The model under review builds one solid part; all positions refer to its coordinate system, in mm. A direction names the side the tool comes from. Give positions to 0.01 mm unless a question says otherwise; leave off trailing zeros. Write each loop counter-clockwise with the first axis right and the second up, starting at its lowest first coordinate (ties: lowest second). Pieces come first, ordered by that corner, then holes. Notation, with made-up numbers: M 86.5,80 L 99.5,80 A17 cw 99.5,105 Z; hole C -15,83 d5. An arc over 180 degrees is marked long. Write each question's results on one line, items separated by ' | '. Start each with the question number.
from build123d import *

# Parameters (mm, degrees)
F0_W     = 112.393752
F0_H     = 112.393752
F1_DEPTH = 50
F2_R     = 20
F3_DEPTH = 30
F2_R_2   = 30
F4_DEPTH = 20


with BuildPart() as f1:
    # F0 (on Top) → F1 (new body)
    with BuildSketch(Plane.XY):
        Rectangle(F0_W, F0_H)
    extrude(amount=F1_DEPTH)

    # F2 (on face) → F3 (cut)
    with BuildSketch(Plane.XY.offset(50)):
        Circle(F2_R)
    extrude(amount=-F3_DEPTH, mode=Mode.SUBTRACT)

    # F2 (on face) → F4 (cut)
    with BuildSketch(Plane.XY.offset(50)):
        with Locations((9.99, 0)):
            Circle(F2_R_2)
        Circle(F2_R, mode=Mode.SUBTRACT)
    extrude(amount=-F4_DEPTH, mode=Mode.SUBTRACT)


solid = f1.part
(1) Add section C-C (x = 9.99). State the section outline as (y, z) points.
(2) Clearance check with flat-ended pins moving along their axes: P1, Ø18, axis at x = 7, y = -6.5, coming from the +Z side; P2, Ø4, axis at x = 31, y = 15, coming from the +Z side. State where each tip first meets the part, or that it passes through.
(3) Add section D-D (y = 23.5). State the section outline as (x, z) points.
(4) Wall thickness on L1, parallel to Y at x = 9.99, z = 40.5; L2, parallel to Y at x = 0, z = 25.75; L3, parallel to Z at x = 7.5, y = -17: over which ranges is each line inside the solid? List them lowest first.
(5) Add section A-A (z = 41.5). State the section outline as (x, y) points.
(6) Machinability: for faces 1 (the cylindrical face through (-19.98, 1.32, 40.14)), 2 (the flat face through (-1, 56.197, 25)), which of the approach directions +Z, -Z, +X, -X, +Y, -Y give a long, thin tool a straight path to every point of the face, cutting with its end or side? Answer none if there is none.
(7) Draft analysis for pull direction Y (two halves, no side actions). For faces 3 (the flat face through (-1, 1, 0)), 4 (the flat face through (-1, -56.197, 25)), 5 (the flat face through (0, 0, 20)), state which applies: pulls with the +Y half, pulls with the -Y half, needs draft (parallel to the pull), parting line crosses it, or undercut.
Calculated:
1) outline: M -56.2,0 L 56.2,0 L 56.2,50 L 30,50 L 30,30 L 17.33,30 L 17.33,20 L -17.33,20 L -17.33,30 L -30,30 L -30,50 L -56.2,50 Z
2) P1: stops at z = 20 | P2: stops at z = 30
3) outline: M -56.2,0 L 56.2,0 L 56.2,50 L 28.64,50 L 28.64,30 L -8.66,30 L -8.66,50 L -56.2,50 Z
4) L1: y = -56.2 to -30, 30 to 56.2 | L2: y = -56.2 to -20, 20 to 56.2 | L3: z = 0 to 20
5) outline: M -56.2,-56.2 L 56.2,-56.2 L 56.2,56.2 L -56.2,56.2 Z; hole C 9.99,0 d60
6) face 1: +Z | face 2: +Z, -Z, +X, -X, +Y
7) face 3: needs draft | face 4: pulls with the -Y half | face 5: undercut
